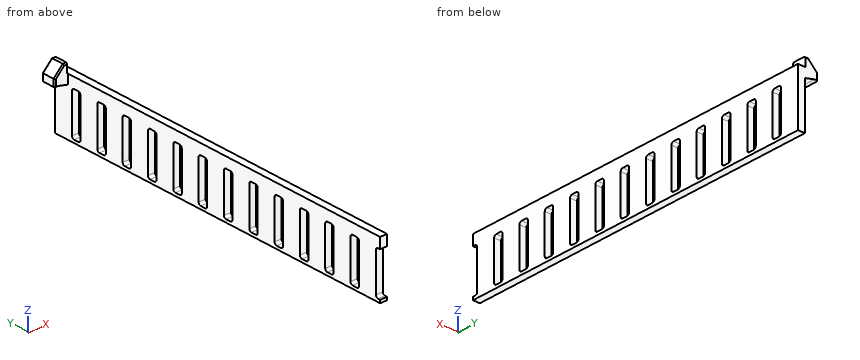
```python
from build123d import *

# Parameters (mm, degrees)
PAD006_DEPTH    = 6
SKETCH014_W     = 3
SKETCH014_H     = 24.25
PAD007_DEPTH    = 148
POCKET007_DEPTH = 3
CHAMFER002_SIZE = 0.5


with BuildPart() as part:
    # Sketch013 (on Face1 of CopyPocket007) → Pad006 (new body)
    with BuildSketch(Plane.XZ.offset(-98)):
        Polygon((-193.75, 37.75), (-197, 37.75), (-197, 41.75), (-198.5, 41.75), (-202.5, 37.75), (-202.5, 34.75), (-201, 34.75), (-197, 33.75), (-196.75, 33.75), (-196.75, 13.5), (-193.75, 13.5), align=None)
    extrude(amount=PAD006_DEPTH)

    # Sketch014 (on Face13 of Pad006) → Pad007 (join)
    with BuildSketch(Plane.XZ.offset(-92)):
        with Locations((-195.25, 25.625)):
            Rectangle(SKETCH014_W, SKETCH014_H)
    extrude(amount=PAD007_DEPTH)

    # Sketch015 (on Face14 of Pad007) → Pocket007 (cut)
    with BuildSketch(Plane(origin=(-196.75, 18, 0), x_dir=(0, -1, 0), z_dir=(-1, 0, 0))):
        with BuildLine():
            Line((-72, 32.25), (-72, 15.75))
            ThreePointArc((-72, 15.75), (-71.7071067812, 15.0428932188), (-71, 14.75))
            Line((-71, 14.75), (-69, 14.75))
            ThreePointArc((-69, 14.75), (-68.2928932188, 15.0428932188), (-68, 15.75))
            Line((-68, 15.75), (-68, 32.25))
            ThreePointArc((-68, 32.25), (-68.2928932188, 32.9571067812), (-69, 33.25))
            Line((-69, 33.25), (-71, 33.25))
            ThreePointArc((-71, 33.25), (-71.7071067812, 32.9571067812), (-72, 32.25))
        make_face()
        with BuildLine():
            Line((-60, 32.2499996536), (-60, 15.7499996536))
            ThreePointArc((-60, 15.7499996536), (-59.7071067812, 15.0428928724), (-59, 14.7499996536))
            Line((-59, 14.7499996536), (-57, 14.7499996536))
            ThreePointArc((-57, 14.7499996536), (-56.2928932188, 15.0428928724), (-56, 15.7499996536))
            Line((-56, 15.7499996536), (-56, 32.2499996536))
            ThreePointArc((-56, 32.2499996536), (-56.2928932188, 32.9571064348), (-57, 33.2499996536))
            Line((-57, 33.2499996536), (-59, 33.2499996536))
            ThreePointArc((-59, 33.2499996536), (-59.7071067812, 32.9571064348), (-60, 32.2499996536))
        make_face()
        with BuildLine():
            Line((-47.9999996732, 32.25), (-47.9999996732, 15.75))
            ThreePointArc((-47.9999996732, 15.75), (-47.7071064544, 15.0428932188), (-46.9999996732, 14.75))
            Line((-46.9999996732, 14.75), (-44.9999996732, 14.75))
            ThreePointArc((-44.9999996732, 14.75), (-44.292892892, 15.0428932188), (-43.9999996732, 15.75))
            Line((-43.9999996732, 15.75), (-43.9999996732, 32.25))
            ThreePointArc((-43.9999996732, 32.25), (-44.292892892, 32.9571067812), (-44.9999996732, 33.25))
            Line((-44.9999996732, 33.25), (-46.9999996732, 33.25))
            ThreePointArc((-46.9999996732, 33.25), (-47.7071064544, 32.9571067812), (-47.9999996732, 32.25))
        make_face()
        with BuildLine():
            Line((-36, 32.25), (-36, 15.75))
            ThreePointArc((-36, 15.75), (-35.7071067812, 15.0428932188), (-35, 14.75))
            Line((-35, 14.75), (-33, 14.75))
            ThreePointArc((-33, 14.75), (-32.2928932188, 15.0428932188), (-32, 15.75))
            Line((-32, 15.75), (-32, 32.25))
            ThreePointArc((-32, 32.25), (-32.2928932188, 32.9571067812), (-33, 33.25))
            Line((-33, 33.25), (-35, 33.25))
            ThreePointArc((-35, 33.25), (-35.7071067812, 32.9571067812), (-36, 32.25))
        make_face()
        with BuildLine():
            Line((-24, 32.25), (-24, 15.75))
            ThreePointArc((-24, 15.75), (-23.7071067812, 15.0428932188), (-23, 14.75))
            Line((-23, 14.75), (-21, 14.75))
            ThreePointArc((-21, 14.75), (-20.2928932188, 15.0428932188), (-20, 15.75))
            Line((-20, 15.75), (-20, 32.25))
            ThreePointArc((-20, 32.25), (-20.2928932188, 32.9571067812), (-21, 33.25))
            Line((-21, 33.25), (-23, 33.25))
            ThreePointArc((-23, 33.25), (-23.7071067812, 32.9571067812), (-24, 32.25))
        make_face()
        with BuildLine():
            Line((-11.9999996732, 32.25), (-11.9999996732, 15.75))
            ThreePointArc((-11.9999996732, 15.75), (-11.7071064544, 15.0428932188), (-10.9999996732, 14.75))
            Line((-10.9999996732, 14.75), (-8.9999996732, 14.75))
            ThreePointArc((-8.9999996732, 14.75), (-8.292892892, 15.0428932188), (-7.9999996732, 15.75))
            Line((-7.9999996732, 15.75), (-7.9999996732, 32.25))
            ThreePointArc((-7.9999996732, 32.25), (-8.292892892, 32.9571067812), (-8.9999996732, 33.25))
            Line((-8.9999996732, 33.25), (-10.9999996732, 33.25))
            ThreePointArc((-10.9999996732, 33.25), (-11.7071064544, 32.9571067812), (-11.9999996732, 32.25))
        make_face()
        with BuildLine():
            Line((0, 32.25), (0, 15.75))
            ThreePointArc((0, 15.75), (0.2928932188, 15.0428932188), (1, 14.75))
            Line((1, 14.75), (3, 14.75))
            ThreePointArc((3, 14.75), (3.7071067812, 15.0428932188), (4, 15.75))
            Line((4, 15.75), (4, 32.25))
            ThreePointArc((4, 32.25), (3.7071067812, 32.9571067812), (3, 33.25))
            Line((3, 33.25), (1, 33.25))
            ThreePointArc((1, 33.25), (0.2928932188, 32.9571067812), (0, 32.25))
        make_face()
        with BuildLine():
            Line((12, 32.25), (12, 15.75))
            ThreePointArc((12, 15.75), (12.2928932188, 15.0428932188), (13, 14.75))
            Line((13, 14.75), (15, 14.75))
            ThreePointArc((15, 14.75), (15.7071067812, 15.0428932188), (16, 15.75))
            Line((16, 15.75), (16, 32.25))
            ThreePointArc((16, 32.25), (15.7071067812, 32.9571067812), (15, 33.25))
            Line((15, 33.25), (13, 33.25))
            ThreePointArc((13, 33.25), (12.2928932188, 32.9571067812), (12, 32.25))
        make_face()
        with BuildLine():
            Line((24.0000003268, 32.25), (24.0000003268, 15.75))
            ThreePointArc((24.0000003268, 15.75), (24.2928935456, 15.0428932188), (25.0000003268, 14.75))
            Line((25.0000003268, 14.75), (27.0000003268, 14.75))
            ThreePointArc((27.0000003268, 14.75), (27.707107108, 15.0428932188), (28.0000003268, 15.75))
            Line((28.0000003268, 15.75), (28.0000003268, 32.25))
            ThreePointArc((28.0000003268, 32.25), (27.707107108, 32.9571067812), (27.0000003268, 33.25))
            Line((27.0000003268, 33.25), (25.0000003268, 33.25))
            ThreePointArc((25.0000003268, 33.25), (24.2928935456, 32.9571067812), (24.0000003268, 32.25))
        make_face()
        with BuildLine():
            Line((36.0000003268, 32.25), (36.0000003268, 15.75))
            ThreePointArc((36.0000003268, 15.75), (36.2928935456, 15.0428932188), (37.0000003268, 14.75))
            Line((37.0000003268, 14.75), (39.0000003268, 14.75))
            ThreePointArc((39.0000003268, 14.75), (39.707107108, 15.0428932188), (40.0000003268, 15.75))
            Line((40.0000003268, 15.75), (40.0000003268, 32.25))
            ThreePointArc((40.0000003268, 32.25), (39.707107108, 32.9571067812), (39.0000003268, 33.25))
            Line((39.0000003268, 33.25), (37.0000003268, 33.25))
            ThreePointArc((37.0000003268, 33.25), (36.2928935456, 32.9571067812), (36.0000003268, 32.25))
        make_face()
        with BuildLine():
            Line((48, 32.25), (48, 15.75))
            ThreePointArc((48, 15.75), (48.2928932188, 15.0428932188), (49, 14.75))
            Line((49, 14.75), (51, 14.75))
            ThreePointArc((51, 14.75), (51.7071067812, 15.0428932188), (52, 15.75))
            Line((52, 15.75), (52, 32.25))
            ThreePointArc((52, 32.25), (51.7071067812, 32.9571067812), (51, 33.25))
            Line((51, 33.25), (49, 33.25))
            ThreePointArc((49, 33.25), (48.2928932188, 32.9571067812), (48, 32.25))
        make_face()
        with BuildLine():
            Line((60.0000003268, 32.25), (60.0000003268, 15.75))
            ThreePointArc((60.0000003268, 15.75), (60.2928935456, 15.0428932188), (61.0000003268, 14.75))
            Line((61.0000003268, 14.75), (63.0000003268, 14.75))
            ThreePointArc((63.0000003268, 14.75), (63.707107108, 15.0428932188), (64.0000003268, 15.75))
            Line((64.0000003268, 15.75), (64.0000003268, 32.25))
            ThreePointArc((64.0000003268, 32.25), (63.707107108, 32.9571067812), (63.0000003268, 33.25))
            Line((63.0000003268, 33.25), (61.0000003268, 33.25))
            ThreePointArc((61.0000003268, 33.25), (60.2928935456, 32.9571067812), (60.0000003268, 32.25))
        make_face()
        with BuildLine():
            Line((72, 32.2499996536), (72, 15.7499996536))
            ThreePointArc((72, 15.7499996536), (72.2928932188, 15.0428928724), (73, 14.7499996536))
            Line((73, 14.7499996536), (75, 14.7499996536))
            ThreePointArc((75, 14.7499996536), (75.7071067812, 15.0428928724), (76, 15.7499996536))
            Line((76, 15.7499996536), (76, 32.2499996536))
            ThreePointArc((76, 32.2499996536), (75.7071067812, 32.9571064348), (75, 33.2499996536))
            Line((75, 33.2499996536), (73, 33.2499996536))
            ThreePointArc((73, 33.2499996536), (72.2928932188, 32.9571064348), (72, 32.2499996536))
        make_face()
    extrude(amount=-POCKET007_DEPTH, mode=Mode.SUBTRACT)

    # Chamfer002
    chamfer002_edges = [part.edges().sort_by_distance(p)[0] for p in [
        (-197.75, 92, 41.75),
        (-200.5, 92, 39.75),
        (-202.5, 92, 36.25),
        (-202.5, 98, 36.25),
        (-200.5, 98, 39.75),
        (-197.75, 98, 41.75),
    ]]
    chamfer(chamfer002_edges, length=CHAMFER002_SIZE)


with BuildPart() as part_1:
    # Body005 placement: moved
    add(part.part.moved(Location((0, 216, 0))))


solid = part_1.part
```
Check sheet for the modelled part. Datum: model origin and axes. Units: mm. Round coordinates to 2 decimals unless told otherwise and drop trailing zeros. Order: outer loops, then holes, each group sorted by start corner. A loop starts at its lowest first (then second) coordinate and runs counter-clockwise, first axis right, second up.
1) Section check A-A (z = 20.75). Give the number of separate pieces and of enclosed holes in the cut face, and give its area (3 significant figures).
2) Go/stop test with flat-tipped pins: pin 1 Ø1.5 at (x, z) = (-195, 27.5) entering from -Y; pin 2 Ø2 at (x, y) = (-195.5, 268) entering from +Z; pin 3 Ø8 at (y, z) = (192, 27.5) entering from -X. Record where each tip stops, or that it passes through.
3) Scan lines: line 1 (Z direction, x = -196.5, y = 199); line 2 (X direction, y = 271.5, z = 22.5); line 3 (Y direction, x = -202, z = 36.75). Record each from-to range of solid material in increasing order.
4) Section check B-B (y = 203). Record the boundary of the cut face in (x, z).
Result:
1. separate pieces: 13
1. enclosed holes: 0
1. area: 312 mm2
2. pin 1: stops at y = 162
2. pin 2: stops at z = 37.75
2. pin 3: stops at x = -196.75
3. line 1: z = 13.5 to 37.75
3. line 2: x = -196.75 to -193.75
3. line 3: y = 308 to 314
4. outline: (-196.75, 13.5) - (-193.75, 13.5) - (-193.75, 37.75) - (-196.75, 37.75) - close
